from build123d import *

# Parameters (mm, degrees)
F0_R     = 33
F0_R_2   = 3.25
F0_R_3   = 20
F0_R_4   = 10
F1_DEPTH = 10
F2_DEPTH = 7


with BuildPart() as f1:
    # F0 (on Front) → F1 (new body)
    with BuildSketch(Plane.XZ):
        Circle(F0_R)
        with Locations((-21.9121137141, -12.5195478067)):
            Circle(F0_R_2, mode=Mode.SUBTRACT)
        with Locations((21.7983033015, -12.7166732237)):
            Circle(F0_R_2, mode=Mode.SUBTRACT)
        Circle(F0_R_3, mode=Mode.SUBTRACT)
        with Locations((0.1138104126, 25.2362210304)):
            Circle(F0_R_2, mode=Mode.SUBTRACT)
        Circle(F0_R_3)
        Circle(F0_R_4, mode=Mode.SUBTRACT)
    extrude(amount=-F1_DEPTH)

    # F0 (on Front) → F2 (join)
    with BuildSketch(Plane.XZ):
        Circle(F0_R_3)
        Circle(F0_R_4, mode=Mode.SUBTRACT)
    extrude(amount=F2_DEPTH)


solid = f1.part
The listing builds one solid part. Answer for the finished solid, in the listing's coordinates (mm). A direction names the side the tool comes from. Give positions to 0.01 mm unless a question says otherwise; leave off trailing zeros. Order: outer loops, then holes, each group sorted by start corner. A loop starts at its lowest first (then second) coordinate and runs counter-clockwise, first axis right, second up. Notation, with made-up numbers: (-22, 73) - (-13, 73) arc R16 ccw to (-13, 96) - close; hole circle Ø1 at (63.25, -38.5). An arc over 180 degrees is marked (long way). One line per item, written item: value. Start each with the question number.
1) A cutting plane is placed at C-C on y = -2.5. Give the vertices of the cut face in (x, z).
2) A cutting plane is placed at A-A on z = 0. Give the vertices of the cut face in (x, y), then the cut area to 3 significant figures.
3) Find the intervals of material crossed by L1, parallel to Z at x = 0, y = 0.25; L2, parallel to Y at x = 28, z = 16; L3, parallel to Z at x = -6.5, y = -0.75, in increasing order.
4) A cutting plane is placed at D-D on x = 0. Give the vertices of the cut face in (y, z).
5) A cutting plane is placed at B-B on x = -8. Give the vertices of the cut face in (y, z).
6) The mould has two halves that part along Z. Classify faces 1 (the face through (-4.336, -3.451, -19.524)), 2 (the face through (18.55, 4.93, -12.57)), 3 (the face through (7, 10, 8)), 4 (the face through (-0.31, 4.93, 28.46)): released by +Z, released by -Z, zero draft, split by the parting line, or undercut.
7) Given pin 1 Ø8.5 at (x, z) = (21.8, -12.72) entering from -Y; pin 2 Ø10 at (x, y) = (5.5, -4.5) entering from -Z; pin 3 Ø4 at (y, z) = (3, 19.5) entering from -X, each flat-ended and moving along its own axis, determine where each tip first touches the part or whether it passes through.
8) A tool of negligible diameter and unlimited length cuts with its end or side. For faces 5 (the face through (30.5, 4.9, -12.6)), 6 (the face through (22, 0, 0)), from which of +Z, -Z, +X, -X, +Y, -Y can it reach the whole face along a straight path? Write none if from no direction.
Answer sheet:
1. outline: circle Ø40 at (0, 0); hole circle Ø20 at (0, 0)
2. outline: (-33, 0) - (-20, 0) - (-20, -7) - (-10, -7) - (-10, 10) - (-33, 10) - close; (10, -7) - (20, -7) - (20, 0) - (33, 0) - (33, 10) - (10, 10) - close
2. area: 600 mm2
3. L1: z = -33 to -10, 10 to 21.99, 28.48 to 33
3. L2: y = 0 to 10
3. L3: z = -18.91 to -7.6, 7.6 to 18.91
4. outline: (-7, -20) - (0, -20) - (0, -33) - (10, -33) - (10, -10) - (-7, -10) - close; (-7, 10) - (10, 10) - (10, 21.99) - (0, 21.99) - (0, 20) - (-7, 20) - close; (0, 28.48) - (10, 28.48) - (10, 33) - (0, 33) - close
5. outline: (-7, -18.33) - (0, -18.33) - (0, -32.02) - (10, -32.02) - (10, -6) - (-7, -6) - close; (-7, 6) - (10, 6) - (10, 32.02) - (0, 32.02) - (0, 18.33) - (-7, 18.33) - close
6. face 1: split by the parting line
6. face 2: undercut
6. face 3: zero draft
6. face 4: undercut
7. pin 1: stops at y = 0
7. pin 2: stops at z = -32.83
7. pin 3: stops at x = -27.98
8. face 5: +Y, -Y
8. face 6: -Y
